Geometry check sheet. Reference: the model listing, model coordinates, mm. A direction names the side the tool comes from. Round coordinates to 2 decimals unless told otherwise and drop trailing zeros. Order: outer loops, then holes, each group sorted by start corner. A loop starts at its lowest first (then second) coordinate and runs counter-clockwise, first axis right, second up. Notation, with made-up numbers: M 71,40 L 107,40 A29 cw 107,75 Z; hole C -3.5,16.5 d6. An arc over 180 degrees is marked long. Answer as a JSON object with one key per item and string values. Group by question number.
```python
from build123d import *

# Parameters (mm, degrees)
F0_W     = 3
F0_H     = 3
F1_DEPTH = 50


with BuildPart() as f1:
    # F0 (on Top) → F1 (new body)
    with BuildSketch(Plane.XY):
        with BuildLine():
            ThreePointArc((-1.5, 4.2426406871), (0, 4.5), (1.5, 4.2426406871))
            Line((1.5, 4.2426406871), (1.5, 6))
            Line((1.5, 6), (-1.5, 6))
            Line((-1.5, 6), (-1.5, 4.2426406871))
        make_face()
        with BuildLine():
            Line((1.5, -6), (1.5, -4.2426406871))
            ThreePointArc((1.5, -4.2426406871), (0, -4.5), (-1.5, -4.2426406871))
            Line((-1.5, -4.2426406871), (-1.5, -6))
            Line((-1.5, -6), (1.5, -6))
        make_face()
        Rectangle(F0_W, F0_H)
        with BuildLine():
            ThreePointArc((-1.5, -4.2426406871), (0, -4.5), (1.5, -4.2426406871))
            Line((1.5, -4.2426406871), (1.5, -1.5))
            Line((1.5, -1.5), (-1.5, -1.5))
            Line((-1.5, -1.5), (-1.5, -4.2426406871))
        make_face()
        with BuildLine():
            Line((1.5, 1.5), (1.5, 4.2426406871))
            ThreePointArc((1.5, 4.2426406871), (0, 4.5), (-1.5, 4.2426406871))
            Line((-1.5, 4.2426406871), (-1.5, 1.5))
            Line((-1.5, 1.5), (1.5, 1.5))
        make_face()
        with BuildLine():
            Line((1.5, 1.5), (4.2426406871, 1.5))
            ThreePointArc((4.2426406871, 1.5), (3.1819805153, 3.1819805153), (1.5, 4.2426406871))
            Line((1.5, 4.2426406871), (1.5, 1.5))
        make_face()
        with BuildLine():
            ThreePointArc((4.2426406871, -1.5), (4.4351935184, -0.7609589043), (4.5, 0))
            ThreePointArc((4.5, 0), (4.4351935184, 0.7609589043), (4.2426406871, 1.5))
            Line((4.2426406871, 1.5), (1.5, 1.5))
            Line((1.5, 1.5), (1.5, -1.5))
            Line((1.5, -1.5), (4.2426406871, -1.5))
        make_face()
        with BuildLine():
            ThreePointArc((1.5, -4.2426406871), (3.1819805153, -3.1819805153), (4.2426406871, -1.5))
            Line((4.2426406871, -1.5), (1.5, -1.5))
            Line((1.5, -1.5), (1.5, -4.2426406871))
        make_face()
        with BuildLine():
            ThreePointArc((-4.2426406871, -1.5), (-3.1819805153, -3.1819805153), (-1.5, -4.2426406871))
            Line((-1.5, -4.2426406871), (-1.5, -1.5))
            Line((-1.5, -1.5), (-4.2426406871, -1.5))
        make_face()
        with BuildLine():
            Line((-1.5, -1.5), (-1.5, 1.5))
            Line((-1.5, 1.5), (-4.2426406871, 1.5))
            ThreePointArc((-4.2426406871, 1.5), (-4.5, 0), (-4.2426406871, -1.5))
            Line((-4.2426406871, -1.5), (-1.5, -1.5))
        make_face()
        with BuildLine():
            Line((-1.5, 1.5), (-1.5, 4.2426406871))
            ThreePointArc((-1.5, 4.2426406871), (-3.1819805153, 3.1819805153), (-4.2426406871, 1.5))
            Line((-4.2426406871, 1.5), (-1.5, 1.5))
        make_face()
        with BuildLine():
            ThreePointArc((-4.2426406871, -1.5), (-4.5, 0), (-4.2426406871, 1.5))
            Line((-4.2426406871, 1.5), (-6, 1.5))
            Line((-6, 1.5), (-6, -1.5))
            Line((-6, -1.5), (-4.2426406871, -1.5))
        make_face()
        with BuildLine():
            ThreePointArc((4.2426406871, 1.5), (4.4351935184, 0.7609589043), (4.5, 0))
            ThreePointArc((4.5, 0), (4.4351935184, -0.7609589043), (4.2426406871, -1.5))
            Line((4.2426406871, -1.5), (6, -1.5))
            Line((6, -1.5), (6, 1.5))
            Line((6, 1.5), (4.2426406871, 1.5))
        make_face()
    extrude(amount=F1_DEPTH)


solid = f1.part
```
1) Sectioned sample at A-A (z = 9.5). Record the boundary of the cut face in (x, y), then the cut area to 3 significant figures.
2) Go/stop test with flat-tipped pins: P1, Ø4, axis at x = 2.5, z = 24, coming from the +Y side; P2, Ø1.9, axis at x = 5, z = 29.5, coming from the +Y side; P3, Ø0.5, axis at x = 5, z = 23.5, coming from the -Y side; P4, Ø1.9, axis at y = 5, z = 20, coming from the -X side. Record where each tip stops, or that it passes through.
3) Thickness scan on line 1 along Y through (x, z) = (5.25, 42.5); line 2 along Y through (x, z) = (2.5, 3). Record the ranges inside material, lowest first. Write a range as [from, to].
4) Release check for a two-part mould opening along Y. For faces 1 (the flat face through (0, -6, 25)), 2 (the flat face through (-6, 0, 25)), 3 (the cylindrical face through (3.202, 3.162, 24.65)) record: +Y half, -Y half, draft (parallel to the pull), parting line (faces both ways), or undercut.
5) Sectioned sample at B-B (x = -2.25). Record the boundary of the cut face in (y, z), then the cut area to 3 significant figures.
6) Set-up check for faces 4 (the flat face through (5, -1.5, 25)), 5 (the flat face through (1.5, 5, 25)), 6 (the flat face through (-1.5, 5, 25)), 7 (the flat face through (-1.5, -5, 25)): record each of +Z, -Z, +X, -X, +Y, -Y from which the full face is reachable in a straight line by a thin tool's end or side.
7) Sectioned sample at C-C (y = 3). Record the boundary of the cut face in (x, z).
Final values:
{
 "1": {"outline": "M -6,-1.5 L -4.24,-1.5 A4.5 ccw -1.5,-4.24 L -1.5,-6 L 1.5,-6 L 1.5,-4.24 A4.5 ccw 4.24,-1.5 L 6,-1.5 L 6,1.5 L 4.24,1.5 A4.5 ccw 1.5,4.24 L 1.5,6 L -1.5,6 L -1.5,4.24 A4.5 ccw -4.24,1.5 L -6,1.5 Z", "area": "82.6 mm^2"},
 "2": {"P1": "stops at y = 6", "P2": "stops at y = 1.96", "P3": "stops at y = -1.5", "P4": "stops at x = -1.96"},
 "3": {"line 1": "y = [-1.5, 1.5]", "line 2": "y = [-3.74, 3.74]"},
 "4": {"face 1": "-Y half", "face 2": "draft", "face 3": "+Y half"},
 "5": {"outline": "M -3.9,0 L 3.9,0 L 3.9,50 L -3.9,50 Z", "area": "390 mm^2"},
 "6": {"face 4": "+Z, -Z, +X, -Y", "face 5": "+Z, -Z, +X, +Y", "face 6": "+Z, -Z, -X, +Y", "face 7": "+Z, -Z, -X, -Y"},
 "7": {"outline": "M -3.35,0 L 3.35,0 L 3.35,50 L -3.35,50 Z"}
}
